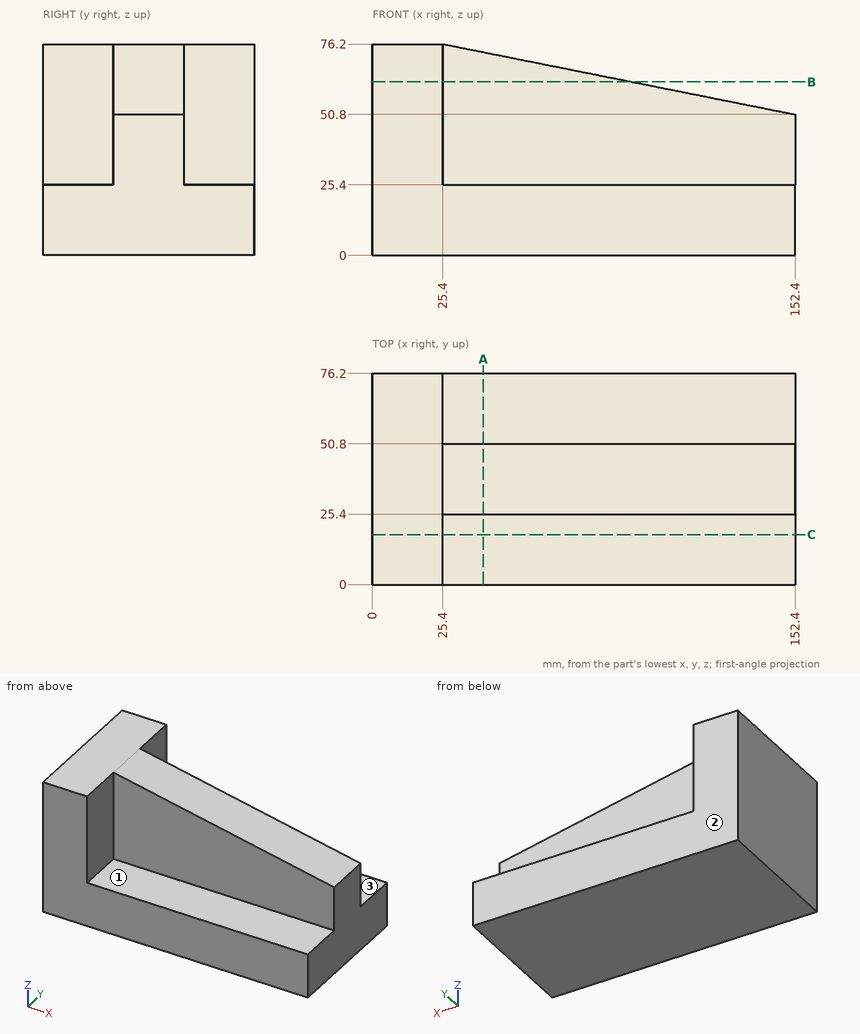
Here's the drawing with two shaded views (mm, measured from the low corner). I have some questions. A direction names the side the tool comes from. Coordinates: 2 decimals unless noted, no trailing zeros. Loops run counter-clockwise (first coordinate to the right, second up) from the corner with the lowest first, then second, coordinate; pieces in that order, holes last. Notation, with made-up numbers: (70, -34) -> (82, -34) arc R25 ccw to (82, 3) -> close; hole circle Ø10 at (-25, -5). An arc over 180 degrees is marked (long way). Answer in a Markdown table with one row per item.
(1) Will these pins go through, and if not, where does the flat tip stop? pin 1 Ø10 at (y, z) = (10, 33.5) entering from +X; pin 2 Ø5 at (x, z) = (40, 35.5) entering from +Y; pin 3 Ø12.5 at (x, y) = (89.5, 10) entering from +Z.
Results found:
| item | result |
|---|---|
| pin 1 | stops at x = 25.4 |
| pin 2 | stops at y = 50.8 |
| pin 3 | stops at z = 25.4 |
(2) Imagine slicing it at B-B (z = 62.5). List the corners of the cut face in (x, y) for me.
Results found:
| item | result |
|---|---|
| outline | (0, 0) -> (25.4, 0) -> (25.4, 25.4) -> (93.9, 25.4) -> (93.9, 50.8) -> (25.4, 50.8) -> (25.4, 76.2) -> (0, 76.2) -> close |
(3) If I drill on probe 1 along Z at (x, y) = (45.5, 9); probe 2 along Y at (x, z) = (99, 28), over which ranges is the centre line in solid material (lowest first)?
Results found:
| item | result |
|---|---|
| probe 1 | z = 0 to 25.4 |
| probe 2 | y = 25.4 to 50.8 |
(4) For the marked faces 1, 2 and 3, which set-ups out of +Z, -Z, +X, -X, +Y, -Y let a thin tool reach every point of the face, with its end or its side?
Results found:
| item | result |
|---|---|
| face 1 | +Z, +X, -Y |
| face 2 | +Z, -Z, +X, -X, +Y |
| face 3 | +Z, +X, +Y |
(5) Imagine slicing it at C-C (y = 18). List the corners of the cut face in (x, z) for me, plus the area to 3 significant figures.
Results found:
| item | result |
|---|---|
| outline | (0, 0) -> (152.4, 0) -> (152.4, 25.4) -> (25.4, 25.4) -> (25.4, 76.2) -> (0, 76.2) -> close |
| area | 5,160 mm^2 |
(6) Imagine slicing it at A-A (x = 40). List the corners of the cut face in (y, z) for me, plus the area to 3 significant figures.
Results found:
| item | result |
|---|---|
| outline | (0, 0) -> (76.2, 0) -> (76.2, 25.4) -> (50.8, 25.4) -> (50.8, 73.28) -> (25.4, 73.28) -> (25.4, 25.4) -> (0, 25.4) -> close |
| area | 3,150 mm^2 |
